```python
from build123d import *

# Parameters (mm, degrees)
SKETCH1_W           = 90
SKETCH1_H           = 11.25
BOSS_EXTRUDE1_DEPTH = 10
LPATTERN1_COUNT     = 4
LPATTERN1_PITCH     = 22.5
SKETCH3_R           = 2
BOSS_EXTRUDE2_DEPTH = 4
DRAFT1_ANGLE        = 1


with BuildPart() as part:
    # Sketch1 → Boss-Extrude1 (new body)
    with BuildSketch(Plane(origin=(0, 0, 0), x_dir=(1, 0, 0), z_dir=(0, 1, 0))):
        with Locations((0, 5.625)):
            Rectangle(SKETCH1_W, SKETCH1_H)
    extrude(amount=BOSS_EXTRUDE1_DEPTH)

    # Sketch2 → Cut-Revolve1 (revolve, cut)
    with BuildSketch(Plane.XY):
        Polygon((-33.75, 8), (-43, 8), (-43, 7), (-35.85, 7), (-35.85, 3), (-36.75, 3), (-35.85, 0), (-33.75, 0), align=None)
    cut_revolve1 = revolve(axis=Axis((-33.75, 16.960495744, 0), (0, -1, 0)), mode=Mode.SUBTRACT)

    # LPattern1: Cut-Revolve1 ×4
    with Locations(*[(i * LPATTERN1_PITCH, 0, 0) for i in range(1, LPATTERN1_COUNT)]):
        add(cut_revolve1, mode=Mode.SUBTRACT)

    # Sketch3 → Boss-Extrude2 (add)
    with BuildSketch(Plane.XY):
        with Locations((-22.5, 4)):
            Circle(SKETCH3_R)
        with Locations((0, 4)):
            Circle(SKETCH3_R)
        with Locations((22.5, 4)):
            Circle(SKETCH3_R)
    extrude(amount=BOSS_EXTRUDE2_DEPTH)

    # Draft1
    draft1_faces = [part.faces().sort_by_distance(p)[0] for p in [
        (20.5, 4, 2),
        (-2, 4, 2),
        (-24.5, 4, 2),
    ]]
    draft(draft1_faces, Plane(origin=(-45, 10, 0), x_dir=(1, 0, 0), z_dir=(0, 0, 1)), DRAFT1_ANGLE)


solid = part.part
```
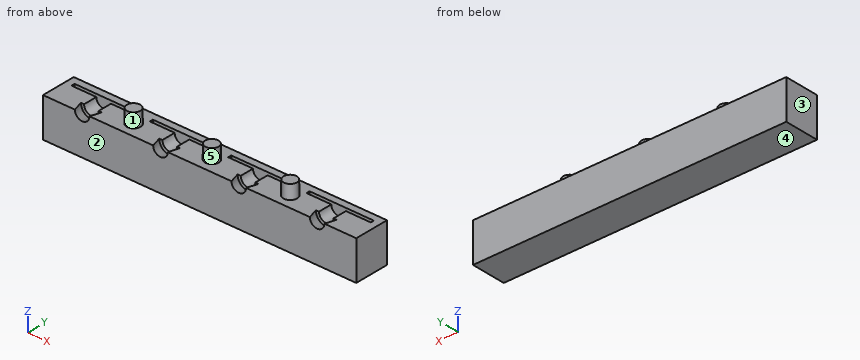
Check sheet for the modelled part. Datum: model origin and axes. Units: mm. Face numbers are marked on the shaded views. A direction names the side the tool comes from. Coordinates: 2 decimals unless noted, no trailing zeros. Order: outer loops, then holes, each group sorted by start corner. A loop starts at its lowest first (then second) coordinate and runs counter-clockwise, first axis right, second up. Notation, with made-up numbers: M 14,42.25 L 63,42.25 A33 cw 63,74.25 Z; hole C 12.25,50 d11. An arc over 180 degrees is marked long. Write each question's results on one line, items separated by ' | '. Start each with the question number.
1. Go/stop test with flat-tipped pins: P1, Ø4, axis at x = 30, z = -9, coming from the -Y side; P2, Ø2, axis at x = 26.5, y = 3, coming from the +Z side; P3, Ø0.9, axis at x = 33.5, z = -1, coming from the -Y side. Record where each tip stops, or that it passes through.
2. Cross-section at A-A on z = -6. Record the cut outline in (x, y), and give its area (3 significant figures).
3. Material ranges on probe 1 along Y at (x, z) = (-28, -2.75); probe 2 along X at (y, z) = (6, -1.25); probe 3 along X at (y, z) = (4.5, 3.25), recorded low to high.
4. Access from +Z, -Z, +X, -X, +Y, -Y to the whole of each face (thin tool, end or side, straight path). Record for the marked faces 1 and 2.
5. Cross-section at C-C on x = -3.5. Record the cut outline in (y, z), and give its area (3 significant figures).
6. Mould release check, pull along X, two halves, no side actions. Record for the marked faces 3, 4 and 5: +X half, -X half, draft (parallel to the pull), parting line (faces both ways), or undercut.
7. Cross-section at B-B on x = 33.75. Record the cut outline in (y, z).
Checks:
1) P1: stops at y = 0 | P2: stops at z = 0 | P3: stops at y = 8
2) outline: M -45,0 L 45,0 L 45,10 L -45,10 Z; hole M -40.79,7 L -26.71,7 L -26.71,8 L -40.79,8 Z; hole M -18.29,7 L -4.21,7 L -4.21,8 L -18.29,8 Z; hole M 4.21,7 L 18.29,7 L 18.29,8 L 4.21,8 Z; hole M 26.71,7 L 40.79,7 L 40.79,8 L 26.71,8 Z | area: 844 mm²
3) probe 1: y = 0 to 7, 8 to 10 | probe 2: x = -45 to -35.44, -32.06 to -12.94, -9.56 to 9.56, 12.94 to 32.06, 35.44 to 45 | probe 3: x = -24.38 to -20.62, -1.88 to 1.88, 20.62 to 24.38
4) face 1: +Z | face 2: +Z, -Z, +X, -X, -Y
5) outline: M 0,-11.25 L 10,-11.25 L 10,0 L 8,0 L 8,-5.05 L 7,-5.05 L 7,0 L 0,0 Z | area: 107 mm²
6) face 3: -X half | face 4: draft | face 5: undercut
7) outline: M 0,-11.25 L 10,-11.25 L 10,0 L 8,0 L 8,-9.25 L 7,-9.25 L 7,-2.1 L 3,-2.1 L 3,-3 L 0,-2.1 Z
